CAD build for the part. Positions are in the model's coordinates, mm. Face numbers are marked on the shaded views. A direction names the side the tool comes from. Give positions to 0.01 mm unless a question says otherwise; leave off trailing zeros. Order: outer loops, then holes, each group sorted by start corner. A loop starts at its lowest first (then second) coordinate and runs counter-clockwise, first axis right, second up.
Item 1: Band-saw the part on A-A on y = 0. Give the cut face in (x, z), plus the area to 3 significant figures.
Item 2: Wall check: L1, parallel to X at y = 0, z = 6.25; L2, parallel to Y at x = -3, z = 8.75. Give the ranges that are in metal, low to high.
Item 3: Flat gauge pins, fed straight in: P1, Ø2.5, axis at y = 20.5, z = 4, coming from the -X side; P2, Ø5, axis at x = -8.5, z = 3, coming from the +Y side; P3, Ø5, axis at x = -7, z = 4.5, coming from the -Y side. Where does each tip first touch, or does it go through?
Item 4: Two-plate mould, pull along X, no slides. Class the marked faces 3 and 4: released by +X, released by -X, zero draft, split by the parting line, or undercut.
Item 5: Which spindle directions (+Z, -Z, +X, -X, +Y, -Y) get a long thin tool onto all of the face, cutting with end or side? Do the marked faces 1 and 2. Say none if no direction does.
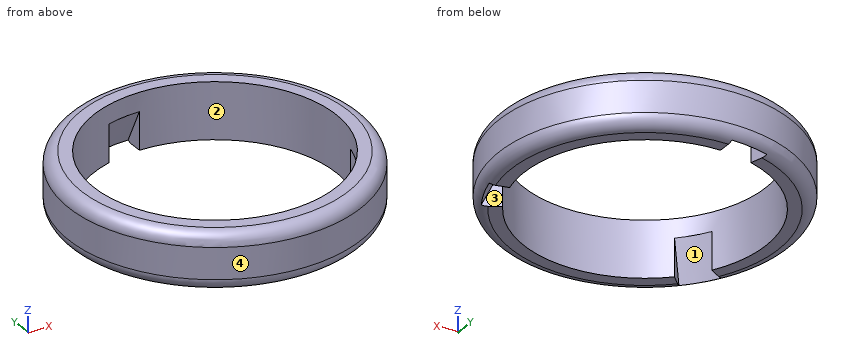
```python
from build123d import *

# Parameters (mm, degrees)
GROOVE_ANGLE    = 16
GROOVE001_ANGLE = 16
GROOVE002_ANGLE = 16


with BuildPart() as part:
    # Sketch027 → Revolution008 (revolve)
    with BuildSketch(Plane.YZ):
        with BuildLine():
            Line((19.3, 0), (21.3, 0))
            ThreePointArc((21.3, 0), (22.714214, 0.585786), (23.3, 2))
            Line((23.3, 2), (23.3, 7))
            ThreePointArc((23.3, 7), (22.714214, 8.414214), (21.3, 9))
            Line((21.3, 9), (19.3, 9))
            Line((19.3, 9), (19.3, 0))
        make_face()
    revolve(axis=Axis((0, 0, 0), (0, 0, 1)))

    # Sketch028 → Groove (revolve, cut)
    with BuildSketch(Plane.YZ):
        Polygon((19.3, 0), (22.3, 0), (19.3, 6), align=None)
    revolve(axis=Axis((0, 0, 0), (0, 0, 1)), revolution_arc=GROOVE_ANGLE, mode=Mode.SUBTRACT)

    # Sketch029 (on DatumPlane) → Groove001 (revolve, cut)
    with BuildSketch(Plane(origin=(0, 0, 0), x_dir=(-0.866025, -0.5, 0), z_dir=(-0.5, 0.866025, 0))):
        Polygon((19.3, 0), (22.3, 0), (19.3, 6), align=None)
    revolve(axis=Axis((0, 0, 0), (0, 0, 1)), revolution_arc=GROOVE001_ANGLE, mode=Mode.SUBTRACT)

    # Sketch047 (on DatumPlane) → Groove002 (revolve, cut)
    with BuildSketch(Plane(origin=(0, 0, 0), x_dir=(0.866025, -0.5, 0), z_dir=(-0.5, -0.866025, 0))):
        Polygon((19.3, 0), (22.3, 0), (19.3, 6), align=None)
    revolve(axis=Axis((0, 0, 0), (0, 0, 1)), revolution_arc=GROOVE002_ANGLE, mode=Mode.SUBTRACT)


solid = part.part
```
The answers:
1. outline: (-23.3, 2) arc R2 ccw to (-21.3, 0) - (-19.3, 0) - (-19.3, 9) - (-21.3, 9) arc R2 ccw to (-23.3, 7) - close; (19.3, 0) - (21.3, 0) arc R2 ccw to (23.3, 2) - (23.3, 7) arc R2 ccw to (21.3, 9) - (19.3, 9) - close
1. area: 68.6 mm2
2. L1: x = -23.3 to -19.3, 19.3 to 23.3
2. L2: y = -22.07 to -19.07, 19.07 to 22.07
3. P1: stops at x = -13.13
3. P2: stops at y = 22.51
3. P3: stops at y = -22.86
4. face 3: undercut
4. face 4: split by the parting line
5. face 1: -Z
5. face 2: +Z, -Z
